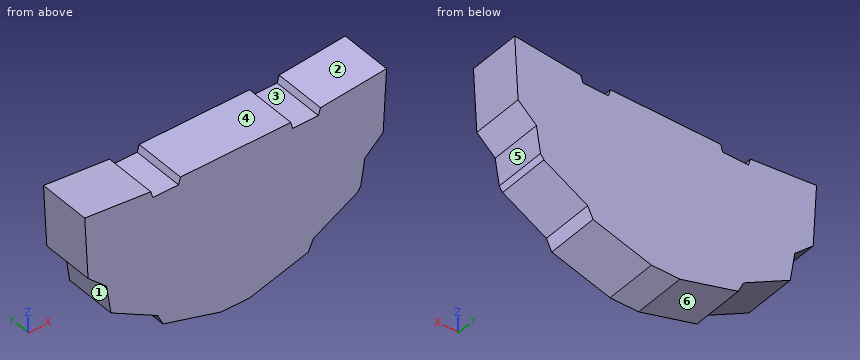
```python
from build123d import *

# Parameters (mm, degrees)
F1_DEPTH = 8
F2_DEPTH = 8
F3_SIZE  = 0.5


with BuildPart() as f1:
    # F0 (on Front) → F1 (new body)
    with BuildSketch(Plane.XZ):
        Polygon((-13.009408, 11.163666), (-23.141133, 12.144796), (-22.627911, 2.564639), (-19.80859, 0), (-19.112445, -4.488478), (-11.951118, -8.457113), (-11.135481, -10.169796), (-2.184, -12.757975), (0, -12.757975), (2.184, -12.757975), (11.135481, -10.169796), (11.951118, -8.457113), (19.112445, -4.488478), (19.80859, 0), (22.627911, 2.564639), (23.141133, 12.144796), (13.009408, 11.163666), (12.689522, 10.10592), (8.754815, 10.10592), (8.461545, 11.163666), (0, 11.163666), (-8.461545, 11.163666), (-8.754815, 10.10592), (-12.689522, 10.10592), align=None)
    extrude(amount=F1_DEPTH)

    # F0 (on Front) → F2 (join)
    with BuildSketch(Plane.XZ):
        Polygon((-13.009408, 11.163666), (-23.141133, 12.144796), (-22.627911, 2.564639), (-19.80859, 0), (-19.112445, -4.488478), (-11.951118, -8.457113), (-11.135481, -10.169796), (-2.184, -12.757975), (0, -12.757975), (2.184, -12.757975), (11.135481, -10.169796), (11.951118, -8.457113), (19.112445, -4.488478), (19.80859, 0), (22.627911, 2.564639), (23.141133, 12.144796), (13.009408, 11.163666), (12.689522, 10.10592), (8.754815, 10.10592), (8.461545, 11.163666), (0, 11.163666), (-8.461545, 11.163666), (-8.754815, 10.10592), (-12.689522, 10.10592), align=None)
    extrude(amount=F2_DEPTH)

    # F3
    f3_edges = [f1.edges().sort_by_distance(p)[0] for p in [
        (19.112445, -4, -4.488478),
    ]]
    chamfer(f3_edges, length=F3_SIZE)


solid = f1.part
```
Work out the finished part from the listing and answer in its coordinate system (mm). Face numbers are marked on the shaded views. A direction names the side the tool comes from. Give positions to 0.01 mm unless a question says otherwise; leave off trailing zeros. Order: outer loops, then holes, each group sorted by start corner. A loop starts at its lowest first (then second) coordinate and runs counter-clockwise, first axis right, second up. Notation, with made-up numbers: M -30,29.25 L 14,29.25 A24 cw 14,44.25 Z; hole C 81.5,-12.75 d6. An arc over 180 degrees is marked long. Return JSON: item names as keys, results as strings.
1) Section A-A, the plane y = -2.25 is taken. Write down the section's boundary in (x, z), plus the area to 3 significant figures.
Resolved:
{"outline": "M -23.14,12.14 L -22.63,2.56 L -19.81,0 L -19.11,-4.49 L -11.95,-8.46 L -11.14,-10.17 L -2.18,-12.76 L 2.18,-12.76 L 11.14,-10.17 L 11.95,-8.46 L 18.68,-4.73 L 19.19,-3.99 L 19.81,0 L 22.63,2.56 L 23.14,12.14 L 13.01,11.16 L 12.69,10.11 L 8.75,10.11 L 8.46,11.16 L -8.46,11.16 L -8.75,10.11 L -12.69,10.11 L -13.01,11.16 Z", "area": "875 mm^2"}
2) Each of these flat-tipped pins is pushed along its axis until it touches: pin 1 (4 mm diameter, centred on y = -1.5, z = 6, fed in from +X); pin 2 (1 mm diameter, centred on y = -2, z = -2.5, fed in from +X); pin 3 (4 mm diameter, centred on y = -3.5, z = -9, fed in from +X); pin 4 (10 mm diameter, centred on x = -8, z = 3.5, fed in from +Y). Where does it stop, or does it pass through?
Resolved:
{"pin 1": "x = 22.92", "pin 2": "x = 19.5", "pin 3": "x = 14.58", "pin 4": "y = 0"}
3) For a pull along X with two mould halves and no side action, classify the marked faces 3, 4, 5 and 6 as +X half, -X half, draft (parallel to the pull), parting line (faces both ways), or undercut.
Resolved:
{"face 3": "undercut", "face 4": "undercut", "face 5": "+X half", "face 6": "-X half"}
4) A tool of negligible diameter and unlimited length cuts with its end or side. For the marked faces 1 and 2, from which of +Z, -Z, +X, -X, +Y, -Y can it reach the whole face along a straight path? Write none if from no direction.
Resolved:
{"face 1": "-Z, -X, +Y, -Y", "face 2": "+Z, +Y, -Y"}
5) Section C-C, the plane z = -9.5 is taken. Write down the section's boundary in (x, y), plus the area to 3 significant figures.
Resolved:
{"outline": "M -11.45,-8 L 11.45,-8 L 11.45,0 L -11.45,0 Z", "area": "183 mm^2"}
6) Straight lines are drawn through the part: line 1 along Z through (x, y) = (0.5, -0.5); line 2 along Z through (x, y) = (-5, -7.5); line 3 along X through (y, z) = (-4, -7). For each, find the intervals that lie inside material, in ascending order. Write a range as [from, to].
Resolved:
{"line 1": "[-12.76, 11.16]", "line 2": "[-11.94, 11.16]", "line 3": "[-14.58, 14.58]"}
7) Section B-B, the plane x = 1.5 is taken. Write down the section's boundary in (y, z).
Resolved:
{"outline": "M -8,-12.76 L 0,-12.76 L 0,11.16 L -8,11.16 Z"}
